```python
from build123d import *

# Parameters (mm, degrees)
BOSS_EXTRU_2_DEPTH      = 8.5
ESQUISSE2_R             = 7.5
BOSS_EXTRU_3_DEPTH      = 2.5
BOSS_EXTRU_4_START      = 1.5
ESQUISSE3_R             = 7.5
BOSS_EXTRU_4_DEPTH      = 1.5
ESQUISSE4_R             = 5
BOSS_EXTRU_5_DEPTH      = 4
ESQUISSE6_R             = 3
ENL_V_MAT_EXTRU_2_DEPTH = 0.1
CONG_4_R                = 1
ENL_V_MAT_EXTRU_3_DEPTH = 20.531001075


with BuildPart() as part:
    # Esquisse1 → Boss.-Extru.2 (new body)
    with BuildSketch(Plane(origin=(0, 0, 0), x_dir=(1, 0, 0), z_dir=(0, 1, 0))):
        Polygon((2.408977243, 1.875974594), (1.487996247, 1.96815707), (1.148248192, 2.829130277), (0.304564016, 2.448472144), (-0.420153034, 3.024222787), (-0.960475898, 2.272721085), (-1.875974594, 2.408977243), (-1.96815707, 1.487996247), (-2.829130277, 1.148248192), (-2.448472144, 0.304564016), (-3.024222787, -0.420153034), (-2.272721085, -0.960475898), (-2.408977243, -1.875974594), (-1.487996247, -1.96815707), (-1.148248192, -2.829130277), (-0.304564016, -2.448472144), (0.420153034, -3.024222787), (0.960475898, -2.272721085), (1.875974594, -2.408977243), (1.96815707, -1.487996247), (2.829130277, -1.148248192), (2.448472144, -0.304564016), (3.024222787, 0.420153034), (2.272721085, 0.960475898), align=None)
    extrude(amount=BOSS_EXTRU_2_DEPTH)

    # Esquisse2 → Boss.-Extru.3 (add)
    with BuildSketch(Plane(origin=(0, 8.5, 0), x_dir=(1, 0, 0), z_dir=(0, 1, 0))):
        with Locations(Location((0, 0, 0), (0, 0, 270))):
            Circle(ESQUISSE2_R)
    extrude(amount=BOSS_EXTRU_3_DEPTH)

    # Esquisse3 → Boss.-Extru.4 (add)
    with BuildSketch(Plane.XZ.offset(BOSS_EXTRU_4_START)):
        with Locations(Location((0, 0, 0), (0, 0, 90))):
            Circle(ESQUISSE3_R)
    extrude(amount=-BOSS_EXTRU_4_DEPTH)

    # Esquisse4 → Boss.-Extru.5 (add)
    with BuildSketch(Plane.XZ.offset(1.5)):
        with Locations(Location((0, 0, 0), (0, 0, 270))):
            Circle(ESQUISSE4_R)
    extrude(amount=BOSS_EXTRU_5_DEPTH)

    # Esquisse6 → Enlèv. mat.-Extru.2 (cut)
    with BuildSketch(Plane.XZ.offset(5.5)):
        with Locations(Location((0, 0, 0), (0, 0, 270))):
            Circle(ESQUISSE6_R)
    extrude(amount=-ENL_V_MAT_EXTRU_2_DEPTH, mode=Mode.SUBTRACT)

    # Congé4
    cong_4_edges = [part.edges().sort_by_distance(p)[0] for p in [
        (0, 11, -7.5),
        (0, -1.5, -7.5),
    ]]
    fillet(cong_4_edges, radius=CONG_4_R)

    # Esquisse7 → Enlèv. mat.-Extru.3 (cut, through all)
    with BuildSketch(Plane.XZ.offset(5.4)):
        with BuildLine():
            Line((-1.048275862, 0), (-1.092437897, -1.169007888))
            ThreePointArc((-1.092437897, -1.169007888), (1.599724111, -0.029711421), (-1.048275862, 1.208767023))
            Line((-1.048275862, 1.208767023), (-1.048275862, 0))
        make_face()
    extrude(amount=-ENL_V_MAT_EXTRU_3_DEPTH, mode=Mode.SUBTRACT)


solid = part.part
```
Part model, mm, in its own coordinate system. A direction names the side the tool comes from. Give positions to 0.01 mm unless a question says otherwise; leave off trailing zeros. Loops run counter-clockwise (first coordinate to the right, second up) from the corner with the lowest first, then second, coordinate; pieces in that order, holes last. Notation, with made-up numbers: M 65.25,89 L 75.25,89 A27 cw 75.25,110 Z; hole C 51,-10.5 d2. An arc over 180 degrees is marked long. Return JSON: item names as keys, results as strings.
1) Flat gauge pins, fed straight in: pin 1 Ø2 at (y, z) = (5, 5.5) entering from +X; pin 2 Ø2 at (y, z) = (5.5, -3.5) entering from +X; pin 3 Ø5 at (y, z) = (1, -3.5) entering from -X. Where does each tip first touch, or does it go through?
Calculated:
{"pin 1": "passes through", "pin 2": "stops at x = 1.28", "pin 3": "stops at x = -7.4"}
2) Drill centre lines: line 1 (Y direction, x = 6.25, z = 0.5); line 2 (X direction, y = -5.35, z = 0); line 3 (Y direction, x = -2.25, z = 3). Where is each one in solid material? Low to high.
Calculated:
{"line 1": "y = -1.5 to 0, 8.5 to 11", "line 2": "x = -5 to -1.05, 1.6 to 5", "line 3": "y = -5.5 to 0, 8.5 to 11"}
3) 3-axis set-ups, long thin cutter, end or side, ignore diameter. For faces 1 (the face through (-4.88, -3.47, 1.08)), 2 (the face through (-0.73, 4.19, 2.64)), 3 (the face through (2.34, 4.19, -1.41)), 4 (the face through (0, 8.5, 3)): which of +Z, -Z, +X, -X, +Y, -Y reach the whole face in a straight line?
Calculated:
{"face 1": "-Y", "face 2": "+Z", "face 3": "+X", "face 4": "none"}
4) Saw through at B-B, the plane y = -2.5. List the corners of the cut face in (x, z), then the cut area to 3 significant figures.
Calculated:
{"outline": "C 0,0 d10; hole M -1.09,-1.17 A1.6 ccw long -1.05,1.21 L -1.05,0 Z", "area": "71.4 mm2"}
5) Saw through at A-A, the plane x = 0. List the corners of the cut face in (y, z).
Calculated:
{"outline": "M -5.5,-5 L -1.5,-5 L -1.5,-6.5 A1 ccw -0.5,-7.5 L 0,-7.5 L 0,-2.69 L 8.5,-2.69 L 8.5,-7.5 L 10,-7.5 A1 ccw 11,-6.5 L 11,-1.6 L -5.4,-1.6 L -5.4,-3 L -5.5,-3 Z; M -5.5,3 L -5.4,3 L -5.4,1.6 L 11,1.6 L 11,6.5 A1 ccw 10,7.5 L 8.5,7.5 L 8.5,2.69 L 0,2.69 L 0,7.5 L -0.5,7.5 A1 ccw -1.5,6.5 L -1.5,5 L -5.5,5 Z"}
6) Saw through at C-C, the plane y = -0.75. List the corners of the cut face in (x, z).
Calculated:
{"outline": "C 0,0 d14.94; hole M -1.09,-1.17 A1.6 ccw long -1.05,1.21 L -1.05,0 Z"}
7) Pull direction Z, two halves, no side cores. Call faces 5 (the face through (1.92, 4.19, 1.95)), 6 (the face through (-1.048, 3, 1)), 7 (the face through (-1.41, 4.19, -2.34)), 8 (the face through (2.64, 4.19, 0.73)): released by +Z, released by -Z, zero draft, split by the parting line, or undercut.
Calculated:
{"face 5": "released by +Z", "face 6": "undercut", "face 7": "released by -Z", "face 8": "undercut"}
